Build history of the part. All positions in model axes, mm. A direction names the side the tool comes from. Round coordinates to 2 decimals unless told otherwise and drop trailing zeros. Loops run counter-clockwise (first coordinate to the right, second up) from the corner with the lowest first, then second, coordinate; pieces in that order, holes last. Notation, with made-up numbers: (-24, 51.5) - (31, 51.5) arc R36 ccw to (31, 90.5) - close; hole circle Ø4 at (23.25, -35). An arc over 180 degrees is marked (long way). One line per question, with ' | ' between items. Start each with the question number.
from build123d import *

# Parameters (mm, degrees)
F0_W     = 145
F0_H     = 75
F0_W_2   = 12
F0_H_2   = 7
F0_R     = 1.5
F0_W_3   = 32
F0_H_3   = 5
F0_W_4   = 90
F0_H_4   = 18
F0_W_5   = 15
F1_DEPTH = 3
F3_DEPTH = 1


with BuildPart() as f1:
    # F0 (on Top) → F1 (new body)
    with BuildSketch(Plane.XY):
        with Locations((72.5, -37.5)):
            Rectangle(F0_W, F0_H)
        with Locations((26, -60.5)):
            Rectangle(F0_W_2, F0_H_2, mode=Mode.SUBTRACT)
        with Locations((44, -60.5)):
            Rectangle(F0_W_2, F0_H_2, mode=Mode.SUBTRACT)
        with Locations((62, -60.5)):
            Rectangle(F0_W_2, F0_H_2, mode=Mode.SUBTRACT)
        with Locations((26, -48.5)):
            Rectangle(F0_W_2, F0_H_2, mode=Mode.SUBTRACT)
        with Locations((44, -48.5)):
            Rectangle(F0_W_2, F0_H_2, mode=Mode.SUBTRACT)
        with Locations((62, -48.5)):
            Rectangle(F0_W_2, F0_H_2, mode=Mode.SUBTRACT)
        with Locations((88, -60.5)):
            Rectangle(F0_W_2, F0_H_2, mode=Mode.SUBTRACT)
        with Locations((88, -48.5)):
            Rectangle(F0_W_2, F0_H_2, mode=Mode.SUBTRACT)
        with Locations((120.617509, -52.318472)):
            Circle(F0_R, mode=Mode.SUBTRACT)
        with Locations((31, -30.5)):
            Rectangle(F0_W_3, F0_H_3, mode=Mode.SUBTRACT)
        with Locations((51.75, -30.71763)):
            Circle(F0_R, mode=Mode.SUBTRACT)
        with Locations((60, -17)):
            Rectangle(F0_W_4, F0_H_4, mode=Mode.SUBTRACT)
        with Locations((72.5, -30.5)):
            Rectangle(F0_W_3, F0_H_3, mode=Mode.SUBTRACT)
        with Locations((97.5, -30.5)):
            Rectangle(F0_W_5, F0_H_3, mode=Mode.SUBTRACT)
        with Locations((120.430524, -29.5)):
            Rectangle(F0_W_2, F0_H_2, mode=Mode.SUBTRACT)
        with Locations((120.617509, -10.455477)):
            Circle(F0_R, mode=Mode.SUBTRACT)
    extrude(amount=F1_DEPTH)

    # F2 (on face) → F3 (join)
    with BuildSketch(Plane.XY.offset(3)):
        with BuildLine():
            Line((13.5, -45), (13, -45))
            ThreePointArc((13, -45), (12.646447, -45.146447), (12.5, -45.5))
            Line((12.5, -45.5), (12.5, -63.5))
            ThreePointArc((12.5, -63.5), (12.646447, -63.853553), (13, -64))
            Line((13, -64), (13.5, -64))
            ThreePointArc((13.5, -64), (13.853553, -63.853553), (14, -63.5))
            Line((14, -63.5), (14, -45.5))
            ThreePointArc((14, -45.5), (13.853553, -45.146447), (13.5, -45))
        make_face()
        with BuildLine():
            Line((101, -45), (100.5, -45))
            ThreePointArc((100.5, -45), (100.146447, -45.146447), (100, -45.5))
            Line((100, -45.5), (100, -63.5))
            ThreePointArc((100, -63.5), (100.146447, -63.853553), (100.5, -64))
            Line((100.5, -64), (101, -64))
            ThreePointArc((101, -64), (101.353553, -63.853553), (101.5, -63.5))
            Line((101.5, -63.5), (101.5, -45.5))
            ThreePointArc((101.5, -45.5), (101.353553, -45.146447), (101, -45))
        make_face()
        with BuildLine():
            Line((75.25, -44.364751), (74.75, -44.364751))
            ThreePointArc((74.75, -44.364751), (74.396447, -44.511198), (74.25, -44.864751))
            Line((74.25, -44.864751), (74.25, -63.5))
            ThreePointArc((74.25, -63.5), (74.396447, -63.853553), (74.75, -64))
            Line((74.75, -64), (75.25, -64))
            ThreePointArc((75.25, -64), (75.603553, -63.853553), (75.75, -63.5))
            Line((75.75, -63.5), (75.75, -44.864751))
            ThreePointArc((75.75, -44.864751), (75.603553, -44.511198), (75.25, -44.364751))
        make_face()
    extrude(amount=F3_DEPTH)


solid = f1.part
1) Saw through at C-C on z = 2.05. State how many separate pieces and enclosed holes the cut face has, and give its area (3 significant figures).
2) Saw through at A-A on x = 51.75. Write the cut outline in (y, z).
3) Drop a flat-ended pin along its axis: pin 1 (1.5 mm diameter, centred on x = 125.5, y = -64.5, fed in from +Z). Give the stop position or say it passes through.
4) Saw through at D-D on y = -41.5. Write the cut outline in (x, z), and give its area (3 significant figures).
5) Saw through at B-B on y = -17. Write the cut outline in (x, z), and give its area (3 significant figures).
6) Wall check: line 1 (X direction, y = -58, z = 3.25); line 2 (Y direction, x = 65, z = 0.75); line 3 (Y direction, x = 97, z = 1.1). Give the ranges that are in metal, low to high. Write a range as [from, to].
7) Tool access for faces 1 (the flat face through (71, -75, 1)), 2 (the flat face through (44, -45, 1)): list every direction of +Z, -Z, +X, -X, +Y, -Y with a clear straight run to the whole face (end or side of a thin tool).
Answer key:
1) separate pieces: 1 | enclosed holes: 16 | area: 8,080 mm²
2) outline: (-75, 0) - (-32.22, 0) - (-32.22, 3) - (-75, 3) - close; (-29.22, 0) - (-26, 0) - (-26, 3) - (-29.22, 3) - close; (-8, 0) - (0, 0) - (0, 3) - (-8, 3) - close
3) pin 1: z = 3
4) outline: (0, 0) - (145, 0) - (145, 3) - (0, 3) - close | area: 435 mm²
5) outline: (0, 0) - (15, 0) - (15, 3) - (0, 3) - close; (105, 0) - (145, 0) - (145, 3) - (105, 3) - close | area: 165 mm²
6) line 1: [12.5, 14], [74.25, 75.75], [100, 101.5] | line 2: [-75, -64], [-57, -52], [-45, -33], [-28, -26], [-8, 0] | line 3: [-75, -33], [-28, -26], [-8, 0]
7) face 1: +Z, -Z, +X, -X, -Y | face 2: +Z, -Z
